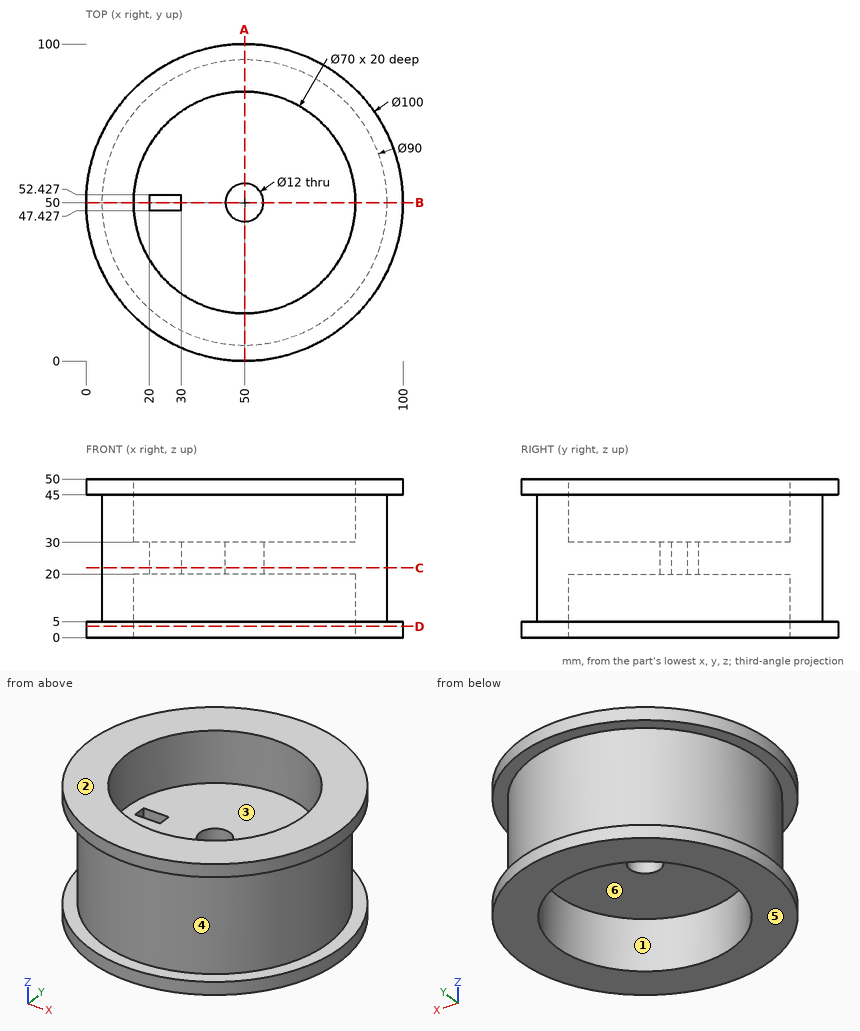
Part print with two shaded views. Sizes in mm from the minimum x, y, z corner. A direction names the side the tool comes from. Round coordinates to 2 decimals unless told otherwise and drop trailing zeros. Loops run counter-clockwise (first coordinate to the right, second up) from the corner with the lowest first, then second, coordinate; pieces in that order, holes last. Notation, with made-up numbers: M -31,48 L -13,48 A25 cw -13,84 Z; hole C 40.5,1 d1. An arc over 180 degrees is marked long. Return JSON: item names as keys, results as strings. Group by question number.
(1) Wall check: probe 1 along Y at (x, z) = (50, 14); probe 2 along Z at (x, y) = (96, 66); probe 3 along Z at (x, y) = (49, 37). Give the ranges that are in metal, low to high. Write a range as [from, to].
(2) Saw through at D-D, the plane z = 3.5. List the corners of the cut face in (x, y), and give its area (3 significant figures).
(3) Tool access for the marked faces 1, 2 and 3: list every direction of +Z, -Z, +X, -X, +Y, -Y with a clear straight run to the whole face (end or side of a thin tool).
(4) Drop flat-ended pins along their axis: P1, Ø11, axis at x = 50, y = 50, coming from the -Z side; P2, Ø4, axis at x = 21.5, y = 38, coming from the -Z side; P3, Ø1.5, axis at y = 49.5, z = 26.5, coming from the -X side; P4, Ø2, axis at y = 53.5, z = 23.5, coming from the +X side. Give the stop position or say it passes through.
(5) Saw through at A-A, the plane x = 50. List the corners of the cut face in (y, z).
(6) Mould opens along Y. For the marked faces 4, 5 and 6 say: +Y half, -Y half, draft (parallel to the pull), parting line (faces both ways), or undercut.
(7) Saw through at C-C, the plane z = 22. List the corners of the cut face in (x, y).
(8) Saw through at B-B, the plane y = 50. List the corners of the cut face in (x, z), and give its area (3 significant figures).
Answer list:
{
 "1": {"probe 1": "[5, 15], [85, 95]", "probe 2": "[0, 5], [45, 50]", "probe 3": "[20, 30]"},
 "2": {"outline": "C 50,50 d100; hole C 50,50 d70", "area": "4,010 mm2"},
 "3": {"face 1": "-Z", "face 2": "+Z, +X, -X, +Y, -Y", "face 3": "+Z"},
 "4": {"P1": "through", "P2": "z = 20", "P3": "x = 5", "P4": "x = 94.93"},
 "5": {"outline": "M 0,0 L 15,0 L 15,20 L 44,20 L 44,30 L 15,30 L 15,50 L 0,50 L 0,45 L 5,45 L 5,5 L 0,5 Z; M 56,20 L 85,20 L 85,0 L 100,0 L 100,5 L 95,5 L 95,45 L 100,45 L 100,50 L 85,50 L 85,30 L 56,30 Z"},
 "6": {"face 4": "parting line", "face 5": "draft", "face 6": "undercut"},
 "7": {"outline": "C 50,50 d90; hole M 20,47.43 L 30,47.43 L 30,52.43 L 20,52.43 Z; hole C 50,50 d12"},
 "8": {"outline": "M 0,0 L 15,0 L 15,20 L 20,20 L 20,30 L 15,30 L 15,50 L 0,50 L 0,45 L 5,45 L 5,5 L 0,5 Z; M 30,20 L 44,20 L 44,30 L 30,30 Z; M 56,20 L 85,20 L 85,0 L 100,0 L 100,5 L 95,5 L 95,45 L 100,45 L 100,50 L 85,50 L 85,30 L 56,30 Z", "area": "1,580 mm2"}
}
